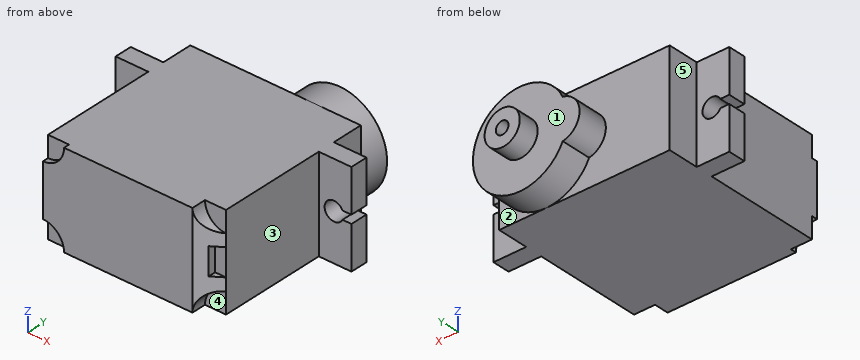
```python
from build123d import *

# Parameters (mm, degrees)
CROQUIS1_W              = 4.5
CROQUIS1_H              = 2.4
CROQUIS1_W_2            = 23.5
CROQUIS1_H_2            = 23.5
SALIENTE_EXTRUIR1_DEPTH = 6.5
SALIENTE_EXTRUIR2_DEPTH = 4.2
CORTAR_EXTRUIR1_REACH   = 27.98
CORTAR_EXTRUIR3_DEPTH   = 0.8
CROQUIS4_5_W            = 1.5
CROQUIS4_5_H            = 3.75
CORTAR_EXTRUIR4_DEPTH   = 2
CORTAR_EXTRUIR5_DEPTH   = 27.219553772
CROQUIS7_R              = 2.425
CROQUIS7_R_2            = 0.875
SALIENTE_EXTRUIR4_DEPTH = 2.85


with BuildPart() as part:
    # Croquis1 → Saliente-Extruir1 (new, symmetric)
    with BuildSketch(Plane.XY):
        with Locations((-14, 6.25)):
            Rectangle(CROQUIS1_W, CROQUIS1_H)
        Rectangle(CROQUIS1_W_2, CROQUIS1_H_2)
        with Locations((14, 6.25)):
            Rectangle(CROQUIS1_W, CROQUIS1_H)
    extrude(amount=SALIENTE_EXTRUIR1_DEPTH, both=True)

    # Croquis2 → Saliente-Extruir2 (add)
    with BuildSketch(Plane(origin=(0, 11.75, 0), x_dir=(1, 0, 0), z_dir=(0, 1, 0))):
        with BuildLine():
            ThreePointArc((-0.636111111, -2.757480007), (11.75, 0), (-0.636111111, 2.757480007))
            ThreePointArc((-0.636111111, 2.757480007), (-2.95, 0), (-0.636111111, -2.757480007))
        make_face()
    extrude(amount=SALIENTE_EXTRUIR2_DEPTH)

    # Croquis3 → Cortar-Extruir1 (cut, up to next)
    with BuildSketch(Plane(origin=(0, 7.45, 0), x_dir=(1, 0, 0), z_dir=(0, 1, 0)), mode=Mode.PRIVATE) as cortar_extruir1_sk1:
        with BuildLine():
            Line((16.25, 0.575), (15.015922382, 0.575))
            ThreePointArc((15.015922382, 0.575), (12.55, 0), (15.015922382, -0.575))
            Line((15.015922382, -0.575), (16.25, -0.575))
            Line((16.25, -0.575), (16.25, 0.575))
        make_face()
    cortar_extruir1_tool1 = extrude(cortar_extruir1_sk1.sketch, amount=-CORTAR_EXTRUIR1_REACH, mode=Mode.PRIVATE) & part.part
    # Croquis3 → Cortar-Extruir1 (cut, up to next)
    with BuildSketch(Plane(origin=(0, 7.45, 0), x_dir=(1, 0, 0), z_dir=(0, 1, 0)), mode=Mode.PRIVATE) as cortar_extruir1_sk2:
        with BuildLine():
            Line((-16.25, 0.575), (-15.015922382, 0.575))
            ThreePointArc((-15.015922382, 0.575), (-12.55, 0), (-15.015922382, -0.575))
            Line((-15.015922382, -0.575), (-16.25, -0.575))
            Line((-16.25, -0.575), (-16.25, 0.575))
        make_face()
    cortar_extruir1_tool2 = extrude(cortar_extruir1_sk2.sketch, amount=-CORTAR_EXTRUIR1_REACH, mode=Mode.PRIVATE) & part.part
    add(cortar_extruir1_tool1.solids().sort_by_distance((14.212834, 7.45, 0))[0], mode=Mode.SUBTRACT)
    add(cortar_extruir1_tool2.solids().sort_by_distance((-14.212834, 7.45, 0))[0], mode=Mode.SUBTRACT)

    # Croquis4 → Cortar-Extruir3 (cut)
    with BuildSketch(Plane.XZ.offset(11.75)):
        with BuildLine():
            Line((-11.75, 6.5), (-11.75, 3.6))
            ThreePointArc((-11.75, 3.6), (-9.699390335, 4.449390335), (-8.85, 6.5))
            Line((-8.85, 6.5), (-11.75, 6.5))
        make_face()
        with BuildLine():
            ThreePointArc((-8.85, -6.5), (-9.699390335, -4.449390335), (-11.75, -3.6))
            Line((-11.75, -3.6), (-11.75, -6.5))
            Line((-11.75, -6.5), (-8.85, -6.5))
        make_face()
    extrude(amount=-CORTAR_EXTRUIR3_DEPTH, mode=Mode.SUBTRACT)

    # Croquis4_5 → Cortar-Extruir4 (cut)
    with BuildSketch(Plane.XZ.offset(11.75)):
        with BuildLine():
            Line((11.75, 6.5), (8.85, 6.5))
            ThreePointArc((8.85, 6.5), (9.699390335, 4.449390335), (11.75, 3.6))
            Line((11.75, 3.6), (11.75, 6.5))
        make_face()
        with BuildLine():
            ThreePointArc((11.75, -3.6), (9.699390335, -4.449390335), (8.85, -6.5))
            Line((8.85, -6.5), (11.75, -6.5))
            Line((11.75, -6.5), (11.75, -3.6))
        make_face()
        with Locations((11, 0)):
            Rectangle(CROQUIS4_5_W, CROQUIS4_5_H)
    extrude(amount=-CORTAR_EXTRUIR4_DEPTH, mode=Mode.SUBTRACT)

    # Croquis6 → Cortar-Extruir5 (cut, through all)
    with BuildSketch(Plane(origin=(0, 0, -6.5), x_dir=(-1, 0, 0), z_dir=(0, 0, -1))):
        Polygon((-11.75, -9.75), (-8.85, -11.75), (-11.75, -11.75), align=None)
    extrude(amount=-CORTAR_EXTRUIR5_DEPTH, mode=Mode.SUBTRACT)

    # Croquis7 → Saliente-Extruir4 (add)
    with BuildSketch(Plane(origin=(0, 15.95, 0), x_dir=(1, 0, 0), z_dir=(0, 1, 0))):
        with Locations(Location((5.25, 0, 0), (0, 0, 270))):
            Circle(CROQUIS7_R)
        with Locations(Location((5.25, 0, 0), (0, 0, 270))):
            Circle(CROQUIS7_R_2, mode=Mode.SUBTRACT)
    extrude(amount=SALIENTE_EXTRUIR4_DEPTH)


solid = part.part
```
Can you work these out from the model? Positions are in its coordinate system, mm. Face numbers are marked on the shaded views. A direction names the side the tool comes from. Give positions to 0.01 mm unless a question says otherwise; leave off trailing zeros. Loops run counter-clockwise (first coordinate to the right, second up) from the corner with the lowest first, then second, coordinate; pieces in that order, holes last. Notation, with made-up numbers: M 37,81.25 L 94,81.25 A25 cw 94,93.25 Z; hole C 88.25,68.5 d8. An arc over 180 degrees is marked long. One line per question, with ' | ' between items. Start each with the question number.
Q1. For the marked faces 1, 2, 3, 4 and 5, which set-ups out of +Z, -Z, +X, -X, +Y, -Y let a thin tool reach every point of the face, with its end or its side?
Q2. If we section it at C-C (y = 15.5): Please give me the cut outline in (x, z).
Q3. If we section it at D-D (x = 0): Please give me the cut outline in (y, z), plus the area to 3 significant figures.
Q4. If we section it at B-B (z = -4.25): Please give me the cut outline in (x, y).
Q5. If we section it at A-A (x = 13.85): Please give me the cut outline in (y, z), plus the area to 3 significant figures.
Q6. If I drill on line 1 (Z direction, x = 13.85, y = 6.5); line 2 (Y direction, x = -1, z = -1.5); line 3 (Y direction, x = -8.5, z = 2.25), over which ranges is the centre line in solid material (lowest first)? Write a range as from..to.
Q7. For pin 1 Ø1.5 at (x, z) = (11, 5) entering from -Y; pin 2 Ø4 at (x, z) = (-0.5, 2.5) entering from +Y; pin 3 Ø5 at (y, z) = (15.5, -3) entering from -X (3 decimals); pin 4 Ø1.6 at (x, z) = (-13.85, 0) entering from +Y, each with a flat end and sliding along its axis, tell me the tip position at first contact or that it passes through.
Computed:
1) face 1: +Y | face 2: -Z, +X, +Y | face 3: +Z, -Z, +X, -Y | face 4: -Z, +X, -Y | face 5: +Z, -Z, -X, +Y
2) outline: M -0.64,-2.76 A6.5 ccw long -0.64,2.76 A2.8 ccw Z
3) outline: M -11.75,-6.5 L 11.75,-6.5 L 11.75,-3.83 L 15.95,-3.83 L 15.95,3.83 L 11.75,3.83 L 11.75,6.5 L -11.75,6.5 Z | area: 338 mm²
4) outline: M -16.25,5.05 L -11.75,5.05 L -11.75,-10.95 L -9.92,-10.95 L -9.92,-11.75 L 8.85,-11.75 L 9.92,-11.01 L 9.92,-9.75 L 11.75,-9.75 L 11.75,5.05 L 16.25,5.05 L 16.25,7.45 L 11.75,7.45 L 11.75,11.75 L 10.17,11.75 L 10.17,15.95 L 0.33,15.95 L 0.33,11.75 L -11.75,11.75 L -11.75,7.45 L -16.25,7.45 Z
5) outline: M 5.05,-6.5 L 7.45,-6.5 L 7.45,-1.3 L 5.05,-1.3 Z; M 5.05,1.3 L 7.45,1.3 L 7.45,6.5 L 5.05,6.5 Z | area: 25.0 mm²
6) line 1: z = -6.5..-1.3, 1.3..6.5 | line 2: y = -11.75..15.95 | line 3: y = -11.75..11.75
7) pin 1: stops at y = -9.75 | pin 2: stops at y = 15.95 | pin 3: stops at x = -2.905 | pin 4: passes through
